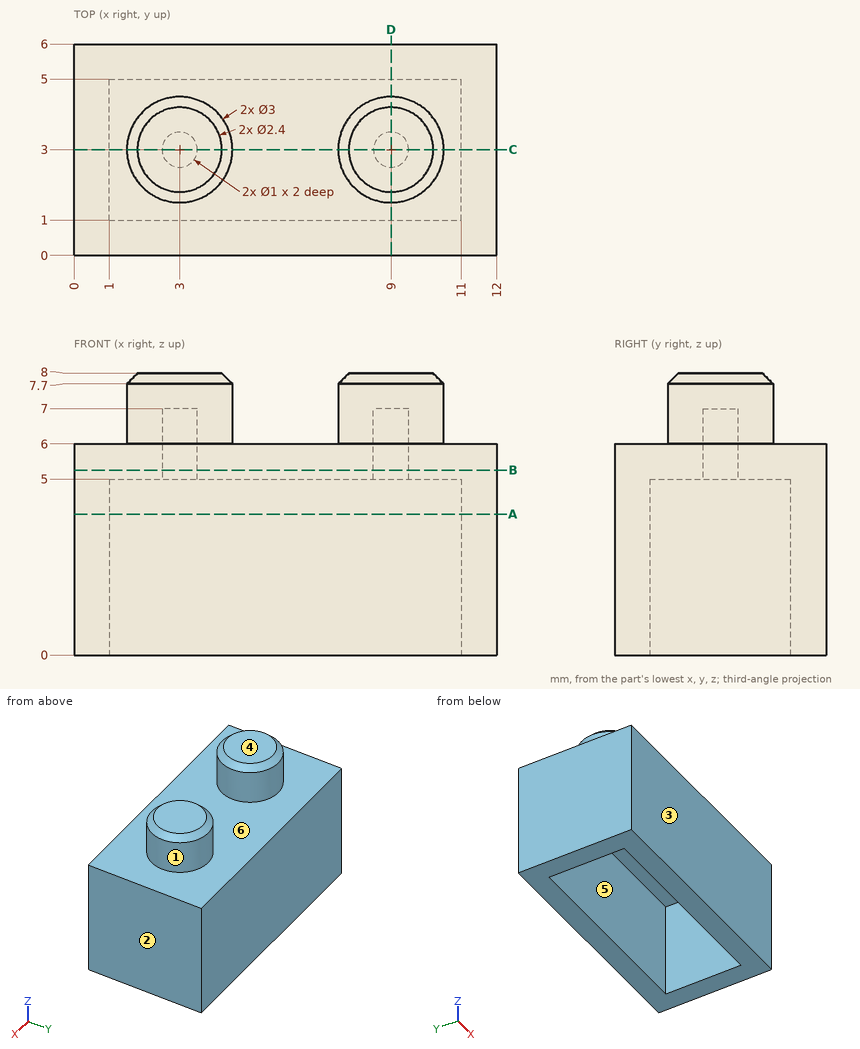
Geometry check sheet. Reference: drawing and pictorial views, mm from the part's lowest x, y, z. A direction names the side the tool comes from. Give positions to 0.01 mm unless a question says otherwise; leave off trailing zeros. Write each loop counter-clockwise with the first axis right and the second up, starting at its lowest first coordinate (ties: lowest second). Pieces come first, ordered by that corner, then holes. Notation, with made-up numbers: (-10, 37) - (40, 37) arc R11 ccw to (40, 56) - close; hole circle Ø6 at (-23.5, 66). An arc over 180 degrees is marked (long way). Put each result on its own line as item: value.
Q1. Scan lines: probe 1 along X at (y, z) = (2.05, 3.5); probe 2 along Y at (x, z) = (8.25, 2.75); probe 3 along X at (y, z) = (3, 5.95). Record each from-to range of solid material in increasing order. Write a range as from..to.
Result:
probe 1: 0..1, 11..12
probe 2: 0..1, 5..6
probe 3: 0..2.5, 3.5..8.5, 9.5..12
Q2. Mould release check, pull along X, two halves, no side actions. Record for the marked faces 1, 2 and 3: released by +X, released by -X, zero draft, split by the parting line, or undercut.
Result:
face 1: undercut
face 2: released by +X
face 3: zero draft
Q3. Section check A-A on z = 4. Record the cut outline in (x, y).
Result:
outline: (0, 0) - (12, 0) - (12, 6) - (0, 6) - close; hole (1, 1) - (11, 1) - (11, 5) - (1, 5) - close
Q4. Depth check by flat-ended pin: P1, Ø3, axis at y = 2.5, z = 3, coming from the -X side; P2, Ø1, axis at x = 1.5, z = 7, coming from the +Y side; P3, Ø1.1, axis at x = 3, y = 3, coming from the -Z side; P4, Ø0.5, axis at x = 9, y = 3, coming from the -Z side. Enter the tip coordinate at first touch or a pass-through.
Result:
P1: x = 0
P2: y = 4.12
P3: z = 5
P4: z = 7
Q5. Section check B-B on z = 5.25. Record the cut outline in (x, y), and give its area (3 significant figures).
Result:
outline: (0, 0) - (12, 0) - (12, 6) - (0, 6) - close; hole circle Ø1 at (3, 3); hole circle Ø1 at (9, 3)
area: 70.4 mm2
Q6. Section check C-C on y = 3. Record the cut outline in (x, z), and give its area (3 significant figures).
Result:
outline: (0, 0) - (1, 0) - (1, 5) - (2.5, 5) - (2.5, 7) - (3.5, 7) - (3.5, 5) - (8.5, 5) - (8.5, 7) - (9.5, 7) - (9.5, 5) - (11, 5) - (11, 0) - (12, 0) - (12, 6) - (10.5, 6) - (10.5, 7.7) - (10.2, 8) - (7.8, 8) - (7.5, 7.7) - (7.5, 6) - (4.5, 6) - (4.5, 7.7) - (4.2, 8) - (1.8, 8) - (1.5, 7.7) - (1.5, 6) - (0, 6) - close
area: 29.8 mm2
Q7. Section check D-D on x = 9. Record the cut outline in (y, z), and give its area (3 significant figures).
Result:
outline: (0, 0) - (1, 0) - (1, 5) - (2.5, 5) - (2.5, 7) - (3.5, 7) - (3.5, 5) - (5, 5) - (5, 0) - (6, 0) - (6, 6) - (4.5, 6) - (4.5, 7.7) - (4.2, 8) - (1.8, 8) - (1.5, 7.7) - (1.5, 6) - (0, 6) - close
area: 19.9 mm2
Q8. Set-up check for the marked faces 4, 5 and 6: record each of +Z, -Z, +X, -X, +Y, -Y from which the full face is reachable in a straight line by a thin tool's end or side.
Result:
face 4: +Z, +X, -X, +Y, -Y
face 5: -Z
face 6: +Z
